Part model, mm, in its own coordinate system. Face numbers are marked on the shaded views. Round coordinates to 2 decimals unless told otherwise and drop trailing zeros. Write each loop counter-clockwise with the first axis right and the second up, starting at its lowest first coordinate (ties: lowest second). Pieces come first, ordered by that corner, then holes. Notation, with made-up numbers: M 83.5,-39.5 L 104.5,-39.5 A25 ccw 104.5,-9.5 Z; hole C -4.75,9.5 d7. An arc over 180 degrees is marked long. Answer as a JSON object with one key per item and string values. Group by question number.
1. Drop flat-ended pins along their axis: pin 1 (3 mm diameter, centred on y = 5, z = 14, fed in from +X); pin 2 (1.5 mm diameter, centred on x = -6.5, y = -5.5, fed in from -Z); pin 3 (1.5 mm diameter, centred on x = 3.5, z = 9.5, fed in from +Y). Give the stop position or say it passes through.
2. Two-plate mould, pull along X, no slides. Class the marked faces 1, 2 and 3: +X half, -X half, draft (parallel to the pull), parting line (faces both ways), or undercut.
3. Drill centre lines: line 1 (X direction, y = 0, z = 4.25); line 2 (Z direction, x = -6, y = -2.25). Where is each one in solid material? Low to high. Write a range as from..to.
4. Band-saw the part on B-B, the plane z = 8.25. Write the cut outline in (x, y).
5. Band-saw the part on A-A, the plane y = 0. Write the cut outline in (x, z).
6. Band-saw the part on D-D, the plane z = 14. Write the cut outline in (x, y), plus the area to 3 significant figures.
from build123d import *

# Parameters (mm, degrees)
F0_W     = 7.62
F0_H     = 11.43
F2_R     = 1.27
F3_R     = 7.366
F4_DEPTH = 12.7


with BuildPart() as f1:
    # F0 (on Right) → F1 (revolve)
    with BuildSketch(Plane.YZ):
        with Locations((3.81, 5.715)):
            Rectangle(F0_W, F0_H)
        Polygon((0, 17.78), (0, 11.43), (7.62, 11.43), (10.16, 11.43), (10.16, 17.78), align=None)
    revolve(axis=Axis((0, 0, 5.715), (0, 0, 1)))

    # F2
    f2_edges = [f1.edges().sort_by_distance(p)[0] for p in [
        (0, -10.16, 11.43),
        (0, -10.16, 17.78),
        (0, 10.16, 14.605),
    ]]
    fillet(f2_edges, radius=F2_R)

    # F3 (on face) → F4 (cut)
    with BuildSketch(Plane(origin=(0, 0, 0), x_dir=(1, 0, 0), z_dir=(0, 0, -1))):
        Circle(F3_R)
    extrude(amount=-F4_DEPTH, mode=Mode.SUBTRACT)


solid = f1.part
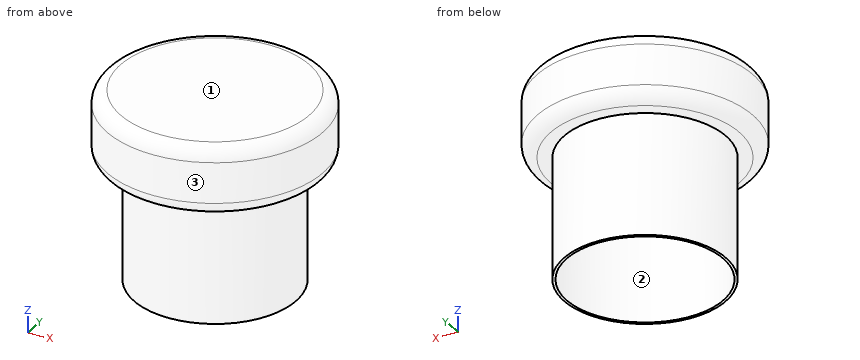
Worked answers:
{
 "1": {"pin 1": "stops at x = 9.54", "pin 2": "stops at z = 11.43", "pin 3": "stops at y = 7.11"},
 "2": {"face 1": "draft", "face 2": "undercut", "face 3": "parting line"},
 "3": {"line 1": "x = -7.62..-7.37, 7.37..7.62", "line 2": "z = 12.7..17.78"},
 "4": {"outline": "C 0,0 d15.24; hole C 0,0 d14.73"},
 "5": {"outline": "M -10.16,12.7 A1.27 ccw -8.89,11.43 L -7.62,11.43 L -7.62,0 L -7.37,0 L -7.37,12.7 L 7.37,12.7 L 7.37,0 L 7.62,0 L 7.62,11.43 L 8.89,11.43 A1.27 ccw 10.16,12.7 L 10.16,16.51 A1.27 ccw 8.89,17.78 L -8.89,17.78 A1.27 ccw -10.16,16.51 Z"},
 "6": {"outline": "C 0,0 d20.32", "area": "324 mm^2"}
}
